Design review of the part shown in the three views and the two pictorial views. Dimensions are in mm from the part's minimum x, y and z. A direction names the side the tool comes from. Coordinates: 2 decimals unless noted, no trailing zeros. Loops run counter-clockwise (first coordinate to the right, second up) from the corner with the lowest first, then second, coordinate; pieces in that order, holes last. Notation, with made-up numbers: (80, -22.5) -> (91, -22.5) arc R29 ccw to (91, 3.5) -> close; hole circle Ø1 at (72, 21). An arc over 180 degrees is marked (long way). Use CSV: the item, a comma, the result in double quotes.
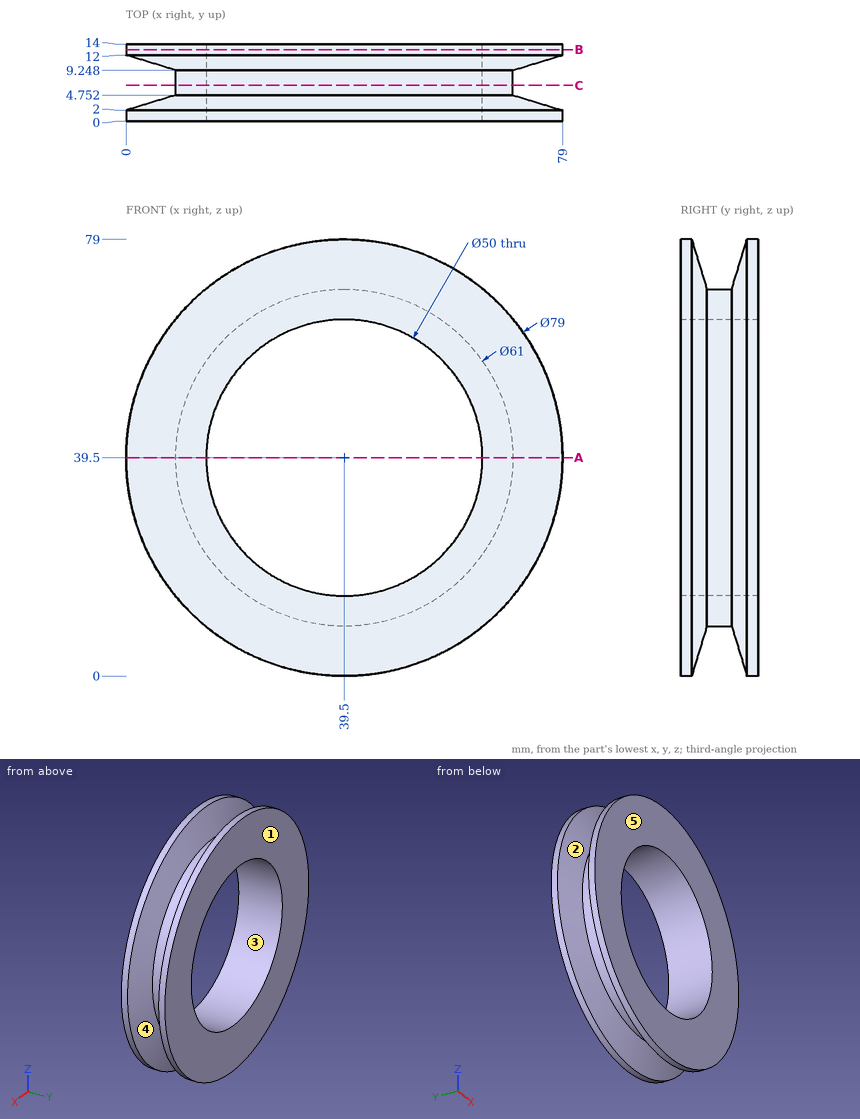
Item 1: To check wall thickness, follow line 1 along Z through (x, y) = (60, 6) (1 decimal); line 2 along Y through (x, z) = (18, 63); line 3 along Z through (x, y) = (28.5, 12.75). State the ranges of each line that lie inside material, in increasing order.
Checked values:
line 1,"16.9 to 25.2, 53.8 to 62.1"
line 2,"0 to 4.34, 9.66 to 14"
line 3,"1.56 to 17.05, 61.95 to 77.44"
Item 2: Add section A-A (z = 39.5). Give the boundary of the cut face in (x, y).
Checked values:
outline,"(0, 0) -> (14.5, 0) -> (14.5, 14) -> (0, 14) -> (0, 12) -> (9, 9.25) -> (9, 4.75) -> (0, 2) -> close; (64.5, 0) -> (79, 0) -> (79, 2) -> (70, 4.75) -> (70, 9.25) -> (79, 12) -> (79, 14) -> (64.5, 14) -> close"
Item 3: Add section B-B (y = 13). Give the boundary of the cut face in (x, z).
Checked values:
outline,"circle Ø79 at (39.5, 39.5); hole circle Ø50 at (39.5, 39.5)"
Item 4: Draft analysis for pull direction Z (two halves, no side actions). For the marked faces 1, 2 and 3, state which applies: pulls with the +Z half, pulls with the -Z half, needs draft (parallel to the pull), parting line crosses it, or undercut.
Checked values:
face 1,"needs draft"
face 2,"parting line crosses it"
face 3,"undercut"
Item 5: Machinability: for the marked faces 4 and 5, which of the approach directions +Z, -Z, +X, -X, +Y, -Y give a long, thin tool a straight path to every point of the face, cutting with its end or side? Answer none if there is none.
Checked values:
face 4,"none"
face 5,"+Z, -Z, +X, -X, -Y"
Item 6: Add section C-C (y = 6.5). Give the boundary of the cut face in (x, z).
Checked values:
outline,"circle Ø61 at (39.5, 39.5); hole circle Ø50 at (39.5, 39.5)"
